Design review of the part built by this model. Coordinates are the model's own, in mm. Round coordinates to 2 decimals unless told otherwise and drop trailing zeros. Order: outer loops, then holes, each group sorted by start corner. A loop starts at its lowest first (then second) coordinate and runs counter-clockwise, first axis right, second up. Notation, with made-up numbers: (51.5, 82.5) - (67.5, 82.5) arc R26 cw to (67.5, 115.5) - close; hole circle Ø1 at (-14, -38.75). An arc over 180 degrees is marked (long way). Use CSV: the item, a comma, the result in double quotes.
from build123d import *

# Parameters (mm, degrees)
F1_DEPTH = 9.5
F3_DEPTH = 19.001


with BuildPart() as f1:
    # F0 (on Right) → F1 (new body, symmetric)
    with BuildSketch(Plane.YZ):
        Polygon((-979.431147, 420), (-979.431147, 0), (0, 0), (0, 900), (-50, 900), (-236.842401, 367.854187), (-250.995365, 372.823452), (-234.431147, 420), align=None)
    extrude(amount=F1_DEPTH, both=True)

    # F2 (on face) → F3 (cut, through all)
    with BuildSketch(Plane(origin=(-9.5, 0, 0), x_dir=(0, -1, 0), z_dir=(-1, 0, 0))):
        Polygon((979.431147, 0), (979.431147, 347.764142), (918.110946, 0), align=None)
        Polygon((960.719799, 351.063457), (979.431147, 347.764142), (979.431147, 420), (972.875172, 420), align=None)
    extrude(amount=-F3_DEPTH, mode=Mode.SUBTRACT)


solid = f1.part
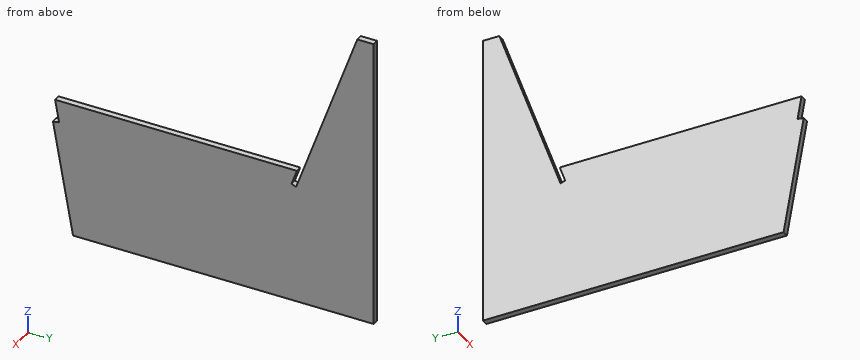
1) To check wall thickness, follow L1, parallel to Z at x = -7.5, y = -436; L2, parallel to Y at x = 7, z = 403; L3, parallel to Y at x = -4.5, z = 176.5. State the ranges of each line that lie inside material, in increasing order. Write a range as from..to.
Data:
L1,"z = 0..420"
L2,"y = -969.88..-240.4, -224.5..0"
L3,"y = -949.23..0"
2) We need section B-B (y = -891.5). Give the boundary of the cut face in (x, z).
Data:
outline,"(-9.5, 0) - (9.5, 0) - (9.5, 420) - (-9.5, 420) - close"
3) Insertion check: pin 1 Ø4 at (x, y) = (-2, -373.5) entering from +Z; pin 2 Ø5 at (x, z) = (-7.5, 236) entering from -Y; pin 3 Ø3 at (x, z) = (4.5, 506.5) entering from +Y. Each pin has a flat end and moves straight along its axis. Give the tip position at first contact, or say it passes through.
Data:
pin 1,"stops at z = 420"
pin 2,"stops at y = -960.16"
pin 3,"stops at y = 0"
4) We need section A-A (x = 2). Give the boundary of the cut face in (y, z).
Data:
outline,"(-979.43, 347.76) - (-918.11, 0) - (0, 0) - (0, 900) - (-50, 900) - (-236.84, 367.85) - (-251, 372.82) - (-234.43, 420) - (-972.88, 420) - (-960.72, 351.06) - close"
5) We need section C-C (z = 472). Give the boundary of the cut face in (x, y).
Data:
outline,"(-9.5, -200.28) - (9.5, -200.28) - (9.5, 0) - (-9.5, 0) - close"
